from build123d import *

# Parameters (mm, degrees)
F0_R     = 35.56
F1_DEPTH = 15.875
F2_SIZE  = 2.54
F3_R     = 35.56
F3_R_2   = 26.67
F4_DEPTH = 6.35


with BuildPart() as f1:
    # F0 (on Right) → F1 (new body, symmetric)
    with BuildSketch(Plane.YZ):
        Circle(F0_R)
        Polygon((-22.868566, 4.947201), (-23.091865, 5.26471), (-22.593373, 7.34102), (-21.776228, 9.313816), (-21.408965, 9.439421), (-18.91785, 9.740089), (-17.24005, 9.589805), (-16.418303, 9.336703), (-15.639718, 8.903017), (-14.711918, 8.811145), (-12.92615, 11.269048), (-13.300231, 12.123061), (-13.95326, 12.72952), (-14.44792, 13.432851), (-15.109308, 14.982086), (-15.593147, 17.444193), (-15.587177, 17.832304), (-13.963484, 19.219065), (-12.142814, 20.334787), (-11.771843, 20.220526), (-9.579779, 18.999523), (-8.310763, 17.891761), (-7.794708, 17.203978), (-7.419732, 16.39549), (-6.723118, 15.775821), (-3.833668, 16.714666), (-3.634351, 17.625449), (-3.806203, 18.499936), (-3.792969, 19.359671), (-3.417421, 21.001798), (-2.361702, 23.278071), (-2.128751, 23.58854), (0, 23.756089), (2.128751, 23.58854), (2.361702, 23.278071), (3.417421, 21.001798), (3.792969, 19.359671), (3.806203, 18.499936), (3.634351, 17.625449), (3.833668, 16.714666), (6.723118, 15.775821), (7.419732, 16.39549), (7.794708, 17.203978), (8.310763, 17.891761), (9.579779, 18.999523), (11.771843, 20.220526), (12.142814, 20.334787), (13.963484, 19.219065), (15.587177, 17.832304), (15.593147, 17.444193), (15.109308, 14.982086), (14.44792, 13.432851), (13.95326, 12.72952), (13.300231, 12.123061), (12.92615, 11.269048), (14.711918, 8.811145), (15.639718, 8.903017), (16.418303, 9.336703), (17.24005, 9.589805), (18.91785, 9.740089), (21.408965, 9.439421), (21.776228, 9.313816), (22.593373, 7.34102), (23.091865, 5.26471), (22.868566, 4.947201), (21.029934, 3.239747), (19.584239, 2.375136), (18.770651, 2.096884), (17.885865, 1.990085), (17.081258, 1.519058), (17.081258, -1.519058), (17.885865, -1.990085), (18.770651, -2.096884), (19.584239, -2.375136), (21.029934, -3.239747), (22.868566, -4.947201), (23.091865, -5.26471), (22.593373, -7.34102), (21.776228, -9.313816), (21.408965, -9.439421), (18.91785, -9.740089), (17.24005, -9.589805), (16.418303, -9.336703), (15.639718, -8.903017), (14.711918, -8.811145), (12.92615, -11.269048), (13.300231, -12.123061), (13.95326, -12.72952), (14.44792, -13.432851), (15.109308, -14.982086), (15.593147, -17.444193), (15.587177, -17.832304), (13.963484, -19.219065), (12.142814, -20.334787), (11.771843, -20.220526), (9.579779, -18.999523), (8.310763, -17.891761), (7.794708, -17.203978), (7.419732, -16.39549), (6.723118, -15.775821), (3.833668, -16.714666), (3.634351, -17.625449), (3.806203, -18.499936), (3.792969, -19.359671), (3.417421, -21.001798), (2.361702, -23.278071), (2.128751, -23.58854), (0, -23.756089), (-2.128751, -23.58854), (-2.361702, -23.278071), (-3.417421, -21.001798), (-3.792969, -19.359671), (-3.806203, -18.499936), (-3.634351, -17.625449), (-3.833668, -16.714666), (-6.723118, -15.775821), (-7.419732, -16.39549), (-7.794708, -17.203978), (-8.310763, -17.891761), (-9.579779, -18.999523), (-11.771843, -20.220526), (-12.142814, -20.334787), (-13.963484, -19.219065), (-15.587177, -17.832304), (-15.593147, -17.444193), (-15.109308, -14.982086), (-14.44792, -13.432851), (-13.95326, -12.72952), (-13.300231, -12.123061), (-12.92615, -11.269048), (-14.711918, -8.811145), (-15.639718, -8.903017), (-16.418303, -9.336703), (-17.24005, -9.589805), (-18.91785, -9.740089), (-21.408965, -9.439421), (-21.776228, -9.313816), (-22.593373, -7.34102), (-23.091865, -5.26471), (-22.868566, -4.947201), (-21.029934, -3.239747), (-19.584239, -2.375136), (-18.770651, -2.096884), (-17.885865, -1.990085), (-17.081258, -1.519058), (-17.081258, 1.519058), (-17.885865, 1.990085), (-18.770651, 2.096884), (-19.584239, 2.375136), (-21.029934, 3.239747), align=None, mode=Mode.SUBTRACT)
    extrude(amount=F1_DEPTH, both=True)

    # F2
    f2_edges = [f1.edges().sort_by_distance(p)[0] for p in [
        (15.875, -35.56, 0),
        (-15.875, -35.56, 0),
    ]]
    chamfer(f2_edges, length=F2_SIZE)

    # F3 (on Right) → F4 (cut, symmetric)
    with BuildSketch(Plane.YZ):
        Circle(F3_R)
        Circle(F3_R_2, mode=Mode.SUBTRACT)
    extrude(amount=F4_DEPTH, both=True, mode=Mode.SUBTRACT)


solid = f1.part
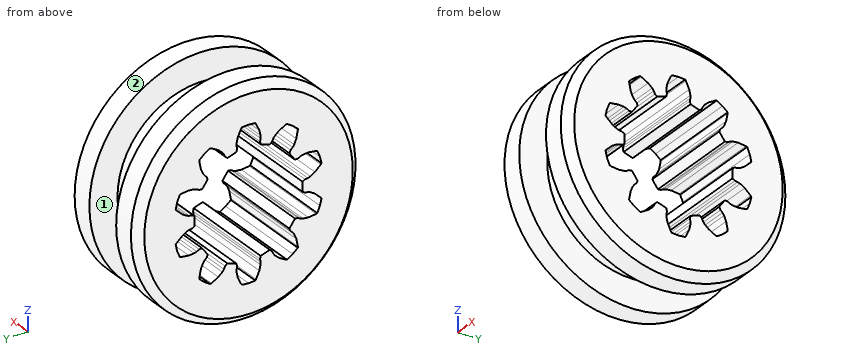
Can you work these out from the model? Positions are in its coordinate system, mm. Face numbers are marked on the shaded views. A direction names the side the tool comes from. Round coordinates to 2 decimals unless told otherwise and drop trailing zeros. Write each loop counter-clockwise with the first axis right and the second up, starting at its lowest first coordinate (ties: lowest second). Pieces come first, ordered by that corner, then holes. Notation, with made-up numbers: (30, -33.5) - (41, -33.5) arc R28 ccw to (41, -5.5) - close; hole circle Ø5 at (86, 36). An arc over 180 degrees is marked (long way). Write each question's results on one line, items separated by ' | '. Start each with the question number.
1) Suppose I cut it at A-A (z = 0). List the corners of the cut face in (x, y) for me (3 decimals).
2) For pin 1 Ø1 at (x, z) = (5.5, 2) entering from +Y; pin 2 Ø1 at (x, y) = (6.5, 21.5) entering from -Z; pin 3 Ø6 at (x, z) = (-5, -10) entering from +Y; pin 4 Ø8 at (y, z) = (-8.5, 11) entering from +X, each with a flat end and sliding along its axis, tell me the tip position at first contact or that it passes through.
3) Which directions (+Z, -Z, +X, -X, +Y, -Y) give clear straight access to the entire face, cutting with the end or side of a thin tool? Please do the marked faces 1 and 2.
4) Please list where these lines run through material, in increasing order: line 1 (Y direction, x = -11, z = 18); line 2 (X direction, y = 14, z = 23) (3 decimals); line 3 (Z direction, x = -6.5, y = 22.5).
Here are the results:
1) outline: (-15.875, -33.02) - (-13.335, -35.56) - (-6.35, -35.56) - (-6.35, -26.67) - (6.35, -26.67) - (6.35, -35.56) - (13.335, -35.56) - (15.875, -33.02) - (15.875, -17.081) - (-15.875, -17.081) - close; (-15.875, 17.081) - (15.875, 17.081) - (15.875, 33.02) - (13.335, 35.56) - (6.35, 35.56) - (6.35, 26.67) - (-6.35, 26.67) - (-6.35, 35.56) - (-13.335, 35.56) - (-15.875, 33.02) - close
2) pin 1: stops at y = 26.63 | pin 2: stops at z = -28.7 | pin 3: stops at y = 34.8 | pin 4: passes through
3) face 1: none | face 2: +X, -X
4) line 1: y = -30.67 to -15.39, -8.43 to -3.71, 3.71 to 8.43, 15.39 to 30.67 | line 2: x = -15.875 to -6.35, 6.35 to 15.875 | line 3: z = -27.54 to -7.57, -4.6 to 4.6, 7.57 to 27.54
